from build123d import *

# Parameters (mm, degrees)
SKETCH1_R               = 10
BOSS_EXTRUDE1_DEPTH     = 18
SKETCH2_R               = 7
CUT_EXTRUDE1_DEPTH      = 15
CUT_EXTRUDE3_DEPTH      = 23.891046285
CUT_EXTRUDE3_DEPTH_BACK = 23.891046285
SKETCH4_R               = 3
FILLET1_R               = 1


with BuildPart() as part:
    # Sketch1 → Boss-Extrude1 (new body)
    with BuildSketch(Plane(origin=(0, 0, 0), x_dir=(1, 0, 0), z_dir=(0, 1, 0))):
        with Locations(Location((0, 0, 0), (0, 0, 270))):
            Circle(SKETCH1_R)
    extrude(amount=BOSS_EXTRUDE1_DEPTH)

    # Sketch2 → Cut-Extrude1 (cut)
    with BuildSketch(Plane(origin=(0, 0, 0), x_dir=(-1, 0, 0), z_dir=(0, -1, 0))):
        with Locations(Location((0, 0, 0), (0, 0, 90))):
            Circle(SKETCH2_R)
    extrude(amount=-CUT_EXTRUDE1_DEPTH, mode=Mode.SUBTRACT)

    # Sketch4 → Cut-Extrude3 (cut, two sides: drawn at the far end of the back side and taken through both)
    with BuildSketch(Plane.XY.offset(-CUT_EXTRUDE3_DEPTH_BACK)):
        with Locations((0, 8)):
            Circle(SKETCH4_R)
    extrude(amount=CUT_EXTRUDE3_DEPTH + CUT_EXTRUDE3_DEPTH_BACK, mode=Mode.SUBTRACT)

    # Fillet1
    fillet1_edges = [part.edges().sort_by_distance(p)[0] for p in [
        (0, 15, 7),
    ]]
    fillet(fillet1_edges, radius=FILLET1_R)


solid = part.part
The listing builds one solid part. Answer for the finished solid, in the listing's coordinates (mm). A direction names the side the tool comes from. Give positions to 0.01 mm unless a question says otherwise; leave off trailing zeros. Write each loop counter-clockwise with the first axis right and the second up, starting at its lowest first coordinate (ties: lowest second). Pieces come first, ordered by that corner, then holes.
1) Section A-A (x = 0) is taken. Write down the section's boundary in (y, z), and give its area (3 significant figures).
2) For a pull along X with two mould halves and no side action, classify faces 1 (the face through (0, 18, 0)), 2 (the face through (2.86, 8.9, 8.14)), 3 (the face through (-3.83, 8.874, 9.237)) as pulls with the +X half, pulls with the -X half, needs draft (parallel to the pull), parting line crosses it, or undercut.
3) Find the intervals of material crossed by L1, parallel to X at y = 3.5, z = 0; L2, parallel to Y at x = 0, z = -8.7, in increasing order.
4) Section D-D (x = -8) is taken. Write down the section's boundary in (y, z).
5) A tool of negligible diameter and unlimited length cuts with its end or side. For faces 4 (the face through (2.86, 8.9, -8.19)), 5 (the face through (-4.259, 6.902, 5.555)), from which of +Z, -Z, +X, -X, +Y, -Y can it reach the whole face along a straight path? Write none if from no direction.
6) Given P1, Ø3.5, axis at x = 0, y = 8, coming from the -Z side; P2, Ø8, axis at y = 4.5, z = 4.5, coming from the +X side; P3, Ø1, axis at x = 2.5, z = -1.5, coming from the -Y side; P4, Ø2, axis at y = 5.5, z = 1.5, coming from the -X side, each flat-ended and moving along its own axis, determine where each tip first touches the part or whether it passes through.
7) Section B-B (z = 0) is taken. Write down the section's boundary in (x, y), and give its area (3 significant figures).
8) Section C-C (y = 8) is taken. Write down the section's boundary in (x, z), and give its area (3 significant figures).
Response:
1. outline: (0, -10) - (5, -10) - (5, -7) - (0, -7) - close; (0, 7) - (5, 7) - (5, 10) - (0, 10) - close; (11, -10) - (18, -10) - (18, 10) - (11, 10) - (11, 7) - (14, 7) arc R1 cw to (15, 6) - (15, -6) arc R1 cw to (14, -7) - (11, -7) - close
1. area: 114 mm2
2. face 1: needs draft
2. face 2: undercut
2. face 3: parting line crosses it
3. L1: x = -10 to -7, 7 to 10
3. L2: y = 0 to 5, 11 to 18
4. outline: (0, -6) - (18, -6) - (18, 6) - (0, 6) - close
5. face 4: +Z, -Z
5. face 5: -Y
6. P1: passes through
6. P2: stops at x = 9.99
6. P3: stops at y = 15
6. P4: stops at x = -9.99
7. outline: (-10, 0) - (-7, 0) - (-7, 14) arc R1 cw to (-6, 15) - (6, 15) arc R1 cw to (7, 14) - (7, 0) - (10, 0) - (10, 18) - (-10, 18) - close
7. area: 150 mm2
8. outline: (-3, -9.54) - (-3, -6.32) arc R7 cw to (-3, 6.32) - (-3, 9.54) arc R10 ccw to start; (3, -9.54) arc R10 ccw to (3, 9.54) - (3, 6.32) arc R7 cw to (3, -6.32) - close
8. area: 123 mm2
